Work out the finished part from the listing and answer in its coordinate system (mm). A direction names the side the tool comes from. Round coordinates to 2 decimals unless told otherwise and drop trailing zeros. Write each loop counter-clockwise with the first axis right and the second up, starting at its lowest first coordinate (ties: lowest second). Pieces come first, ordered by that corner, then holes. Notation, with made-up numbers: M 46,15 L 67,15 A17 ccw 67,24 Z; hole C -4,-21 d6. An arc over 180 degrees is marked long. One line per item, written item: value. Start each with the question number.
Q1. Find section A-A (z = 4.4). Write down the section's boundary in (x, y), and give its area (3 significant figures).
Q2. The mould has two halves that part along Y. Classify faces 1 (the flat face through (50, -100, 3)), 2 (the flat face through (55, -23, 0)), 3 (the cylindrical face through (48.26, 99.97, 3.04)), 4 (the cylindrical face through (14, 23, 3)): released by +Y, released by -Y, zero draft, split by the parting line, or undercut.
Q3. Consider probe 1 along X at (y, z) = (-78, 2.4); probe 2 along Y at (x, z) = (27, 5.85); probe 3 along X at (y, z) = (-32, 0.8). Determine where each line is inside the solid, lowest interval first.
Q4. Find section B-B (x = 50). Write down the section's boundary in (y, z), and give its area (3 significant figures).
Q5. Find section D-D (y = -16). Write down the section's boundary in (x, z).
Q6. A tool of negligible diameter and unlimited length cuts with its end or side. For faces 5 (the flat face through (76, -53, 3)), 6 (the flat face through (55, -23, 6)), 7 (the flat face through (24, -54, 3)), from which of +Z, -Z, +X, -X, +Y, -Y can it reach the whole face along a straight path? Write none if from no direction.
Q7. Find section C-C (y = 71). Write down the section's boundary in (x, z), and give its area (3 significant figures).
Q8. Given pin 1 Ø4 at (x, y) = (27, -94) entering from -Z; pin 2 Ø1.8 at (y, z) = (-60, 2.5) entering from -X; pin 3 Ø2 at (x, z) = (16, 5) entering from +Y; pin 4 Ø3 at (y, z) = (-61, 3) entering from +X, each flat-ended and moving along its own axis, determine where each tip first touches the part or whether it passes through.
from build123d import *

# Parameters (mm, degrees)
ESQUISSE1_W             = 100
ESQUISSE1_H             = 100
BOSS_EXTRU_1_DEPTH      = 6
ESQUISSE2_R             = 45
ENL_V_MAT_EXTRU_1_DEPTH = 142.548578234
ESQUISSE3_W             = 100
ESQUISSE3_H             = 100
BOSS_EXTRU_2_DEPTH      = 6
ESQUISSE4_W             = 24
ESQUISSE4_H             = 100
ENL_V_MAT_EXTRU_2_DEPTH = 6
ESQUISSE5_R             = 1.5
ENL_V_MAT_EXTRU_3_DEPTH = 142.548578234
ENL_V_MAT_EXTRU_4_DEPTH = 142.548578234
CHANFREIN1_SIZE         = 14.962611718


with BuildPart() as part:
    # Esquisse1 → Boss.-Extru.1 (new body)
    with BuildSketch(Plane.XY):
        with Locations((50, 50)):
            Rectangle(ESQUISSE1_W, ESQUISSE1_H)
    extrude(amount=BOSS_EXTRU_1_DEPTH)

    # Esquisse2 → Enlèv. mat.-Extru.1 (cut, through all)
    with BuildSketch(Plane.XY.offset(6)):
        with Locations((50, 50)):
            Circle(ESQUISSE2_R)
    extrude(amount=-ENL_V_MAT_EXTRU_1_DEPTH, mode=Mode.SUBTRACT)

    # Esquisse3 → Boss.-Extru.2 (add)
    with BuildSketch(Plane.XY.offset(6)):
        with Locations((50, -50)):
            Rectangle(ESQUISSE3_W, ESQUISSE3_H)
    extrude(amount=-BOSS_EXTRU_2_DEPTH)

    # Esquisse4 → Enlèv. mat.-Extru.2 (cut)
    with BuildSketch(Plane.XY.offset(6)):
        with Locations((12, -50)):
            Rectangle(ESQUISSE4_W, ESQUISSE4_H)
        with Locations((88, -50)):
            Rectangle(ESQUISSE4_W, ESQUISSE4_H)
    extrude(amount=-ENL_V_MAT_EXTRU_2_DEPTH, mode=Mode.SUBTRACT)

    # Esquisse5 → Enlèv. mat.-Extru.3 (cut, through all)
    with BuildSketch(Plane.XY.offset(6)):
        with Locations((27, -78)):
            Circle(ESQUISSE5_R)
        with Locations((27, -94)):
            Circle(ESQUISSE5_R)
        with Locations(Location((73, -94, 0), (0, 0, 180))):
            Circle(ESQUISSE5_R)
        with Locations(Location((73, -78, 0), (0, 0, 180))):
            Circle(ESQUISSE5_R)
    extrude(amount=-ENL_V_MAT_EXTRU_3_DEPTH, mode=Mode.SUBTRACT)

    # Esquisse6 → Enlèv. mat.-Extru.4 (cut, through all)
    with BuildSketch(Plane.XY.offset(6)):
        with BuildLine():
            Line((76, 7.291686992), (76, 0))
            Line((76, 0), (101, 0))
            Line((101, 0), (101, 101))
            Line((101, 101), (-1, 101))
            Line((-1, 101), (-1, 0))
            Line((-1, 0), (24, 0))
            Line((24, 0), (24, 7.291686992))
            ThreePointArc((24, 7.291686992), (50, 100), (76, 7.291686992))
        make_face()
    extrude(amount=-ENL_V_MAT_EXTRU_4_DEPTH, mode=Mode.SUBTRACT)

    # Chanfrein1
    # the kernel refuses this chamfer: 14.962611718, 5 mm, written as the material it adds along each edge
    with BuildSketch(Plane(origin=(76, 7.291686992, 6), x_dir=(0.8254797465203109, 0.564431739083446, 0), z_dir=(0, 0, -1))) as chanfrein1_piece_1:
        with BuildLine():
            Line((5.28690795, 0), (-CHANFREIN1_SIZE * 0.564431739076, CHANFREIN1_SIZE * 0.825479746509))
            Line((-CHANFREIN1_SIZE * 0.564431739076, CHANFREIN1_SIZE * 0.825479746509), (0, 0))
            ThreePointArc((0, 0), (2.867154561, 0.069426966), (5.28690795, 0))
        make_face()
    extrude(amount=6)
    with BuildSketch(Plane(origin=(24, 7.291686992, 6), x_dir=(-0.8254797465203098, 0.5644317390834476, 0), z_dir=(0, 0, -1))) as chanfrein1_piece_2:
        with BuildLine():
            Line((5.28690795, 0), (-CHANFREIN1_SIZE * 0.564431739076, -CHANFREIN1_SIZE * 0.825479746509))
            Line((-CHANFREIN1_SIZE * 0.564431739076, -CHANFREIN1_SIZE * 0.825479746509), (0, 0))
            ThreePointArc((0, 0), (2.867154561, -0.069426966), (5.28690795, 0))
        make_face()
    extrude(amount=6)


solid = part.part
The answers:
1. outline: M 19.64,10.28 L 24,-7.67 L 24,-100 L 76,-100 L 76,-7.67 L 80.36,10.28 A50 ccw long Z; hole C 50,50 d90; hole C 27,-94 d3; hole C 27,-78 d3; hole C 73,-94 d3; hole C 73,-78 d3
1. area: 6,850 mm2
2. face 1: released by -Y
2. face 2: zero draft
2. face 3: split by the parting line
2. face 4: undercut
3. probe 1: 24 to 25.5, 28.5 to 71.5, 74.5 to 76
3. probe 2: -100 to -95.5, -92.5 to -79.5, -76.5 to 11.32, 88.68 to 94.4
3. probe 3: 24 to 76
4. outline: M -100,0 L 5,0 L 5,6 L -100,6 Z; M 95,0 L 100,0 L 100,6 L 95,6 Z
4. area: 660 mm2
5. outline: M 24,0 L 76,0 L 76,6 L 24,6 Z
6. face 5: +Z, -Z, +X, -Y
6. face 6: +Z, +X, -X, +Y, -Y
6. face 7: +Z, -Z, -X, -Y
7. outline: M 4.62,0 L 10.2,0 L 10.2,6 L 4.62,6 Z; M 89.8,0 L 95.38,0 L 95.38,6 L 89.8,6 Z
7. area: 66.9 mm2
8. pin 1: z = 0
8. pin 2: x = 24
8. pin 3: y = 87.56
8. pin 4: x = 76
